Part model, mm, in its own coordinate system. A direction names the side the tool comes from. Round coordinates to 2 decimals unless told otherwise and drop trailing zeros. Order: outer loops, then holes, each group sorted by start corner. A loop starts at its lowest first (then second) coordinate and runs counter-clockwise, first axis right, second up. Notation, with made-up numbers: (59.5, 20.25) - (118.5, 20.25) arc R7 ccw to (118.5, 30.25) - close; hole circle Ø6 at (-27, -26). An arc over 180 degrees is marked (long way). Return JSON: item names as keys, results as strings. Group by question number.
Item 1: Probe probe 1 along X at (y, z) = (22, 7); probe 2 along Y at (x, z) = (1.5, 7.5); probe 3 along X at (y, z) = (32.5, 3.25) (3 decimals). List the from-to ranges inside material, lowest first.
Item 2: Saw through at C-C on z = -1.25. List the corners of the cut face in (x, y).
Item 3: Saw through at B-B on y = 13.5. List the corners of the cut face in (x, z).
Item 4: Two-plate mould, pull along X, no slides. Class faces 6 (the face through (7.62, 19, 6)), 7 (the face through (0.128, -6.221, -1.005)), 8 (the face through (-10.73, 32.91, 5.08)): released by +X, released by -X, zero draft, split by the parting line, or undercut.
Item 5: Drop flat-ended pins along their axis: pin 1 (4 mm diameter, centred on x = 5.5, y = 7, fed in from -Z); pin 2 (1.2 mm diameter, centred on x = -10.5, y = 30, fed in from -Z); pin 3 (1.3 mm diameter, centred on x = 0.5, z = 8, fed in from -Y). Give the stop position or say it passes through.
Item 6: Tool access for faces 1 (the face through (-9.494, 24.159, 1.274)), 2 (the face through (10, 31, 1.029)), 3 (the face through (0, 30.226, 7)), 4 (the face through (6.58, -2.82, 2.19)), 5 (the face through (0.128, -4.513, 4.107)): list every direction of +Z, -Z, +X, -X, +Y, -Y with a clear straight run to the whole face (end or side of a thin tool).
```python
from build123d import *

# Parameters (mm, degrees)
F1_R      = 1.7859375
F2_DEPTH  = 3.96875
F3_DEPTH  = 9.128125
F4_START  = 9.128125
F0_R      = 1.7859375
F4_DEPTH  = 2.38125
F7_DEPTH  = 11.509375
F6_W      = 15.24
F6_H      = 21.336
F8_DEPTH  = 9.2536280605
F9_R      = 6.35
F11_DEPTH = 10.4116969269
F12_SIZE2 = 4.7625
F12_SIZE  = 1.5875


# Not quite as in the source:
# - a feature names something its author has since deleted; it is built from what else it names


with BuildPart() as f2:
    # F1 (on Right) → F2 (new body, symmetric)
    with BuildSketch(Plane.YZ):
        with BuildLine():
            Line((-3.4820551441, -0.7959792641), (-2.7800674169, -3.8668632517))
            ThreePointArc((-2.7800674169, -3.8668632517), (2.1727097341, -4.2380111682), (4.7625, 0))
            Line((4.7625, 0), (4.7625, 3.571875))
            Line((4.7625, 3.571875), (0, 3.571875))
            ThreePointArc((0, 3.571875), (-2.7929759621, 2.2265615399), (-3.4820551441, -0.7959792641))
        make_face()
        Circle(F1_R, mode=Mode.SUBTRACT)
    extrude(amount=F2_DEPTH, both=True)

    # F1 (on Right) → F3 (join, symmetric)
    with BuildSketch(Plane.YZ):
        with BuildLine():
            Line((-6.9643447844, -2.8750519268), (-5.4621269675, -2.3617314805))
            Line((-5.4621269675, -2.3617314805), (-4.8504655451, -6.2830637627))
            Line((-4.8504655451, -6.2830637627), (-3.8175156986, -5.077588394))
            Line((-3.8175156986, -5.077588394), (-2.7800674169, -3.8668632517))
            Line((-2.7800674169, -3.8668632517), (-3.4820551441, -0.7959792641))
            ThreePointArc((-3.4820551441, -0.7959792641), (-2.7929759621, 2.2265615399), (0, 3.571875))
            Line((0, 3.571875), (4.7625, 3.571875))
            ThreePointArc((4.7625, 3.571875), (5.2274679849, 4.6944070151), (6.35, 5.159375))
            Line((6.35, 5.159375), (6.35, 9.2526280605))
            ThreePointArc((6.35, 9.2526280605), (1.5941526376, 8.3066312028), (-2.4376600757, 5.6126600757))
            Line((-2.4376600757, 5.6126600757), (-5.0921494321, 4.6325641503))
            Line((-5.0921494321, 4.6325641503), (-3.9164474257, 3.5658490795))
            Line((-3.9164474257, 3.5658490795), (-7.0531168828, 1.134330772))
            Line((-7.0531168828, 1.134330772), (-5.4984652486, 0.8130605645))
            Line((-5.4984652486, 0.8130605645), (-6.9643447844, -2.8750519268))
        make_face()
    extrude(amount=F3_DEPTH, both=True)

    # F0 (on Right) → F4 (join)
    with BuildSketch(Plane.YZ.offset(F4_START)):
        with BuildLine():
            ThreePointArc((-2.4376600757, 5.6126600757), (-4.1582937893, 3.0375497444), (-4.7625, 0))
            ThreePointArc((-4.7625, 0), (0, -4.7625), (4.7625, 0))
            Line((4.7625, 0), (4.7625, 3.571875))
            ThreePointArc((4.7625, 3.571875), (5.2274679849, 4.6944070151), (6.35, 5.159375))
            Line((6.35, 5.159375), (6.35, 9.2526280605))
            ThreePointArc((6.35, 9.2526280605), (1.5941526376, 8.3066312028), (-2.4376600757, 5.6126600757))
        make_face()
        Circle(F0_R, mode=Mode.SUBTRACT)
    extrude(amount=F4_DEPTH)


with BuildPart() as f5_1:
    # F5: instance of F2
    add(f2.part.mirror(Plane.YZ))


with BuildPart() as f2_1:
    add(f2.part)

    add(f5_1.part)  # F7 merges F5_1
    # F0 (on Right) → F7 (join, symmetric)
    with BuildSketch(Plane.YZ):
        with BuildLine():
            Line((35.3293530643, 9.2526280605), (6.35, 9.2526280605))
            Line((6.35, 9.2526280605), (6.35, 5.159375))
            ThreePointArc((6.35, 5.159375), (14.3027763595, 4.3544032669), (21.9329443326, 1.9721421521))
            ThreePointArc((21.9329443326, 1.9721421521), (24.1912770347, 1.2670543743), (26.5450934892, 1.0288035264))
            Line((26.5450934892, 1.0288035264), (35.3293530643, 1.0288035264))
            Line((35.3293530643, 1.0288035264), (35.3293530643, 9.2526280605))
        make_face()
    extrude(amount=F7_DEPTH, both=True)

    # F6 (on Top) → F8 (cut, through all)
    with BuildSketch(Plane.XY):
        with Locations((0, 19.558)):
            Rectangle(F6_W, F6_H)
    extrude(amount=F8_DEPTH, mode=Mode.SUBTRACT)

    # F9
    f9_edges = [f2_1.edges().sort_by_distance(p)[0] for p in [
        (-7.62, 30.226, 5.140716),
        (7.62, 30.226, 5.140716),
        (7.62, 8.89, 7.16532),
        (-7.62, 8.89, 7.16532),
    ]]
    fillet(f9_edges, radius=F9_R)

    # F10 (on face) → F11 (cut, through all)
    with BuildSketch(Plane(origin=(0, 35.3293530643, 0), x_dir=(-1, 0, 0), z_dir=(0, 1, 0))):
        with BuildLine():
            Line((-7.62, 1.0288035264), (7.62, 1.0288035264))
            ThreePointArc((7.62, 1.0288035264), (0, 4.8388035264), (-7.62, 1.0288035264))
        make_face()
    extrude(amount=-F11_DEPTH, mode=Mode.SUBTRACT)

    # F12
    f12_edges = [f2_1.edges().sort_by_distance(p)[0] for p in [
        (11.509375, 35.329353, 5.140716),
        (-11.509375, 35.329353, 5.140716),
        (0, 35.329353, 9.252628),
    ]]
    f12_side = f2_1.faces().sort_by_distance((0, 35.329353, 5.838802))[0]
    chamfer(f12_edges, length=F12_SIZE, length2=F12_SIZE2, reference=f12_side)


solid = f2_1.part
```
Filled in:
{
 "1": {"probe 1": "x = -11.51 to -7.62, 7.62 to 11.51", "probe 2": "y = -0.01 to 8.89, 30.22 to 35.33", "probe 3": "x = -10.865 to -5.267, 5.267 to 10.865"},
 "2": {"outline": "(-11.51, -4.6) - (-9.13, -4.6) - (-9.13, -6.32) - (9.13, -6.32) - (9.13, -4.6) - (11.51, -4.6) - (11.51, -1.28) - (9.13, -1.28) - (9.13, -3.38) - (3.97, -3.38) - (3.97, -1.28) - (-3.97, -1.28) - (-3.97, -3.38) - (-9.13, -3.38) - (-9.13, -1.28) - (-11.51, -1.28) - close; (-11.51, 1.28) - (-9.13, 1.28) - (-9.13, 4.6) - (-11.51, 4.6) - close; (-3.97, 1.28) - (3.97, 1.28) - (3.97, 4.6) - (-3.97, 4.6) - close; (9.13, 1.28) - (11.51, 1.28) - (11.51, 4.6) - (9.13, 4.6) - close"},
 "3": {"outline": "(-11.51, 4.51) - (-7.38, 4.51) - (-7.38, 9.25) - (-11.51, 9.25) - close; (7.38, 4.51) - (11.51, 4.51) - (11.51, 9.25) - (7.38, 9.25) - close"},
 "4": {"face 6": "undercut", "face 7": "zero draft", "face 8": "released by -X"},
 "5": {"pin 1": "stops at z = 4.41", "pin 2": "stops at z = 1.03", "pin 3": "stops at y = -0.26"},
 "6": {"face 1": "-Z, +X, -X", "face 2": "-Z, +X, -X, +Y", "face 3": "+Z, -Z", "face 4": "none", "face 5": "+X, -X, -Y"}
}
